from build123d import *

# Parameters (mm, degrees)
F2_R     = 5
F3_DEPTH = 30
F4_W     = 12.7017059222
F4_H     = 7
F5_DEPTH = 5.5
F6_W     = 11.5470053838
F6_H     = 10
F7_DEPTH = 2
F9_DEPTH = 10
F10_R    = 1


with BuildPart() as f3:
    # F2 (on face) → F3 (new body)
    with BuildSketch(Plane(origin=(0, 0, 0), x_dir=(0.8660254038, 0, -0.5), z_dir=(-0.5, 0, -0.8660254038))):
        with Locations((5, 0)):
            Circle(F2_R)
    extrude(amount=-F3_DEPTH)

    # F4 (on Front) → F5 (cut, symmetric)
    with BuildSketch(Plane.XZ):
        with Locations((6.3508529611, -1.5)):
            Rectangle(F4_W, F4_H)
    extrude(amount=F5_DEPTH, both=True, mode=Mode.SUBTRACT)

    # F6 (on face) → F7 (join)
    with BuildSketch(Plane(origin=(0, 0, 2), x_dir=(1, 0, 0), z_dir=(0, 0, -1))):
        with Locations((6.9282032303, 0)):
            Rectangle(F6_W, F6_H)
    extrude(amount=F7_DEPTH)

    # F8 (on face) → F9 (cut)
    with BuildSketch(Plane(origin=(15, 0, 25.9807621135), x_dir=(0.8660254038, 0, -0.5), z_dir=(0.5, 0, 0.8660254038))):
        with BuildLine():
            Line((6.6, 2.6), (3.4, 2.6))
            ThreePointArc((3.4, 2.6), (2.6928932188, 2.3071067812), (2.4, 1.6))
            Line((2.4, 1.6), (2.4, -1.6))
            ThreePointArc((2.4, -1.6), (2.6928932188, -2.3071067812), (3.4, -2.6))
            Line((3.4, -2.6), (6.6, -2.6))
            ThreePointArc((6.6, -2.6), (7.3071067812, -2.3071067812), (7.6, -1.6))
            Line((7.6, -1.6), (7.6, 1.6))
            ThreePointArc((7.6, 1.6), (7.3071067812, 2.3071067812), (6.6, 2.6))
        make_face()
    extrude(amount=-F9_DEPTH, mode=Mode.SUBTRACT)

    # F10
    f10_edges = [f3.edges().sort_by_distance(p)[0] for p in [
        (15, 0, 25.980762),
    ]]
    fillet(f10_edges, radius=F10_R)


solid = f3.part
Geometry: final body of the model. Coordinates: model frame, mm. A direction names the side the tool comes from. Coordinates: 2 decimals unless noted, no trailing zeros. One line per question, with ' | ' between items. Start each with the question number.
(1) First-contact query: pin 1 (5.5 mm diameter, centred on x = 8.5, y = -2.5, fed in from +Z); pin 2 (3 mm diameter, centred on x = 6.5, z = 10, fed in from +Y); pin 3 (2 mm diameter, centred on y = 0.5, z = 0.5, fed in from +X). Flat tips, straight axial feed; report the tip coordinate or a pass-through.
(2) Reachability of faces 1 (the flat face through (12.702, 0, 1)), 2 (the flat face through (7, -5, 1)), 3 (the flat face through (7, 5, 1)), 4 (the cylindrical face through (14.86, -2.3, 20.37)), 5 (the flat face through (2, 4, 2)) from +Z, -Z, +X, -X, +Y, -Y: full face, straight path, thin tool, end or side. Return the list, or none.
(3) Ray query, L1, parallel to X at y = -1.75, z = 15.25; L2, parallel to X at y = 0.75, z = 19.5; L3, parallel to Z at x = 12.25, y = 2.75. Return the intervals inside material, ascending. Write a range as from..to.
(4) Draft query along Y for faces 6 (the flat face through (17, 2.6, 19)), 7 (the cylindrical face through (18.86, -2.31, 18.06)), 8 (the flat face through (2, -4, 2)), 9 (the cylindrical face through (7.738, -0.22, 13.393)). Return one class per face: +Y half, -Y half, draft (parallel to the pull), parting line (faces both ways), or undercut.
Here are the results:
1) pin 1: z = 18.7 | pin 2: y = 4.09 | pin 3: x = 12.7
2) face 1: -Z, +X, +Y, -Y | face 2: +Z, -Z, +X, -X, -Y | face 3: +Z, -Z, +X, -X, +Y | face 4: none | face 5: +Z, -X, +Y
3) L1: 9.17..13.59, 17.57..19.99 | L2: 11.32..14.03, 20.03..22.74 | L3: 0..2, 2.87..19.57
4) face 6: undercut | face 7: undercut | face 8: draft | face 9: parting line
